The model under review builds one solid part; all positions refer to its coordinate system, in mm. Face numbers are marked on the shaded views. A direction names the side the tool comes from. Coordinates: 2 decimals unless noted, no trailing zeros. Order: outer loops, then holes, each group sorted by start corner. A loop starts at its lowest first (then second) coordinate and runs counter-clockwise, first axis right, second up. Notation, with made-up numbers: (-8.5, 50) -> (-2.5, 50) arc R21 ccw to (-2.5, 69) -> close; hole circle Ø5 at (47, 36). An arc over 180 degrees is marked (long way). Use CSV: the item, a comma, the result in double quotes. Start each with the question number.
```python
from build123d import *

# Parameters (mm, degrees)
EXTRUSION1_DEPTH                                = 10
ESQUISSE2_R                                     = 20
EXTRUSION2_DEPTH                                = 12
ESQUISSE3_W                                     = 82
ESQUISSE3_H                                     = 10
EXTRUSION3_DEPTH                                = 37
CONG_1_R                                        = 12
CHAMBRAGE_POUR_VIS_T_TE_CYLINDRIQUE_D           = 11
CHAMBRAGE_POUR_VIS_T_TE_CYLINDRIQUE_CBORE_D     = 22
CHAMBRAGE_POUR_VIS_T_TE_CYLINDRIQUE_CBORE_DEPTH = 1
D_GAGEMENT_M1_61_D                              = 20
NERVURE1_REACH                                  = 77.987
ESQUISSE9_WALL_W                                = 194.58156294
ESQUISSE9_WALL_H                                = 10
CHANFREIN1_SIZE                                 = 1


with BuildPart() as part:
    # Esquisse1 → Extrusion1 (new body)
    with BuildSketch(Plane(origin=(0, 0, 0), x_dir=(0, 0, -1), z_dir=(1, 0, 0))):
        with BuildLine():
            Line((-41, 58), (41, 58))
            Line((41, 58), (41, 48))
            Line((41, 48), (18.539491779, -7.502482561))
            ThreePointArc((18.539491779, -7.502482561), (0, -20), (-18.539491779, -7.502482561))
            Line((-18.539491779, -7.502482561), (-41, 48))
            Line((-41, 48), (-41, 58))
        make_face()
    extrude(amount=-EXTRUSION1_DEPTH)

    # Esquisse2 → Extrusion2 (add)
    with BuildSketch(Plane(origin=(0, 0, 0), x_dir=(0, 0, -1), z_dir=(1, 0, 0))):
        Circle(ESQUISSE2_R)
    extrude(amount=-EXTRUSION2_DEPTH)

    # Esquisse3 → Extrusion3 (add)
    with BuildSketch(Plane.ZY.offset(10)):
        with Locations((0, 53)):
            Rectangle(ESQUISSE3_W, ESQUISSE3_H)
    extrude(amount=-EXTRUSION3_DEPTH)

    # Congé1
    cong_1_edges = [part.edges().sort_by_distance(p)[0] for p in [
        (27, 53, -41),
        (27, 53, 41),
    ]]
    fillet(cong_1_edges, radius=CONG_1_R)

    # Chambrage pour vis à tête cylindrique à 6 pans creux (ou vis CHC) M41 (through all)
    with Locations(Plane.XZ.offset(-48)):
        with Locations((15, 29), (15, -29)):
            CounterBoreHole(CHAMBRAGE_POUR_VIS_T_TE_CYLINDRIQUE_D / 2, CHAMBRAGE_POUR_VIS_T_TE_CYLINDRIQUE_CBORE_D / 2, CHAMBRAGE_POUR_VIS_T_TE_CYLINDRIQUE_CBORE_DEPTH)

    # Dégagement M1.61 (through all)
    with Locations(Plane.ZY.offset(12)):
        with Locations((0, 0)):
            Hole(D_GAGEMENT_M1_61_D / 2)

    # Esquisse9 wall → Nervure1 (add, up to next)
    with BuildSketch(Plane(origin=(12.5, 32, 0), x_dir=(-0.615644041972, -0.788024373725, 0), z_dir=(0.788024373725, -0.615644041972, 0)), mode=Mode.PRIVATE) as nervure1_sk1:
        Rectangle(ESQUISSE9_WALL_W, ESQUISSE9_WALL_H)
    nervure1_tool1 = extrude(nervure1_sk1.sketch, amount=-NERVURE1_REACH, mode=Mode.PRIVATE) - part.part
    add(nervure1_tool1.solids().sort_by_distance((12.5, 32, 0))[0])

    # Chanfrein1
    chanfrein1_edges = [part.edges().sort_by_distance(p)[0] for p in [
        (0, 0, 10),
        (-12, 0, 10),
    ]]
    chamfer(chanfrein1_edges, length=CHANFREIN1_SIZE)


solid = part.part
```
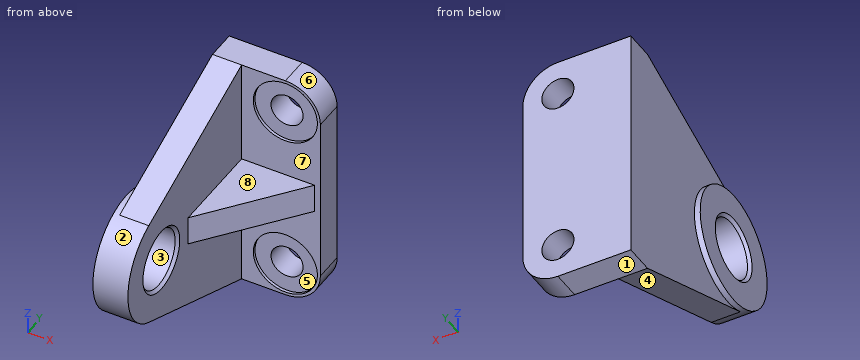
Q1. Add section B-B, the plane y = 0. State the section outline as (x, z) points, then the cut area to 3 significant figures.
Q2. To check wall thickness, follow probe 1 along Z at (x, y) = (18, 49.5); probe 2 along X at (y, z) = (17.5, -10); probe 3 along Y at (x, z) = (3.5, 35). State the ranges of each line that lie inside material, in increasing order.
Q3. For the marked faces 5, 6, 7 and 8, list the 3-axis set-ups (+Z, -Z, +X, -X, +Y, -Y) from which the entire face can be reached by the end or side of a thin tool; tool diameter is ignored.
Q4. Draft analysis for pull direction Y (two halves, no side actions). For the marked faces 1, 2, 3 and 4, state which applies: +Y half, -Y half, draft (parallel to the pull), parting line (faces both ways), or undercut.
Q5. Add section A-A, the plane z = 0. State the section outline as (x, y) points.
Q6. Add section C-C, the plane x = 17. State the section outline as (y, z) points, then the cut area to 3 significant figures.
Q7. Clearance check with flat-ended pins moving along their axes: pin 1 Ø20 at (x, y) = (7, 27.5) entering from -Z; pin 2 Ø10 at (x, y) = (5.5, 14.5) entering from +Z; pin 3 Ø8 at (x, z) = (12.5, 12.5) entering from -Y; pin 4 Ø6.5 at (x, z) = (13.5, 33) entering from -Y. State where each tip first meets the part, or that it passes through.
Q8. Add section D-D, the plane y = 44. State the section outline as (x, z) points (3 decimals).
Answer block:
1,outline,"(-12, -20) -> (-10, -20) -> (-10, -21.58) -> (0, -21.58) -> (0, -11) -> (-1, -10) -> (-11, -10) -> (-12, -11) -> close; (-12, 11) -> (-11, 10) -> (-1, 10) -> (0, 11) -> (0, 21.58) -> (-10, 21.58) -> (-10, 20) -> (-12, 20) -> close"
1,area,"270 mm²"
2,probe 1,"z = -40.62 to -33.61, -24.39 to 24.39, 33.61 to 40.62"
2,probe 2,"x = -10 to 0"
2,probe 3,"y = 48 to 58"
3,face 5,"-Y"
3,face 6,"+Z, +X, +Y, -Y"
3,face 7,"+X, -Y"
3,face 8,"+Z, +X, -Y"
4,face 1,"draft"
4,face 2,"parting line"
4,face 3,"undercut"
4,face 4,"-Y half"
5,outline,"(-12, -20) -> (0, -20) -> (0, -11) -> (-1, -10) -> (-11, -10) -> (-12, -11) -> close; (-12, 11) -> (-11, 10) -> (-1, 10) -> (0, 11) -> (0, 16) -> (25, 48) -> (27, 48) -> (27, 58) -> (-10, 58) -> (-10, 20) -> (-12, 20) -> close"
6,outline,"(37.76, -5) -> (48, -5) -> (48, -18.18) -> (49, -18.18) -> (49, -23.88) -> (58, -23.88) -> (58, 23.88) -> (49, 23.88) -> (49, 18.18) -> (48, 18.18) -> (48, 5) -> (37.76, 5) -> close; (48, -40.83) -> (58, -40.83) -> (58, -34.12) -> (49, -34.12) -> (49, -39.82) -> (48, -39.82) -> close; (48, 39.82) -> (49, 39.82) -> (49, 34.12) -> (58, 34.12) -> (58, 40.83) -> (48, 40.83) -> close"
6,area,"691 mm²"
7,pin 1,"stops at z = -35.59"
7,pin 2,"passes through"
7,pin 3,"stops at y = 48"
7,pin 4,"stops at y = 49"
8,outline,"(-10, -39.381) -> (0, -39.381) -> (0, -5) -> (21.875, -5) -> (21.875, 5) -> (0, 5) -> (0, 39.381) -> (-10, 39.381) -> close"
